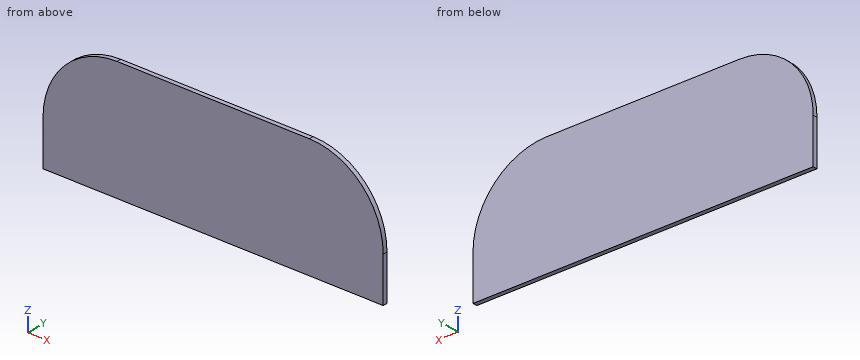
```python
from build123d import *

# Parameters (mm, degrees)
F1_DEPTH = 0.3


with BuildPart() as f1:
    # F0 (on Front) → F1 (new body)
    with BuildSketch(Plane.XZ):
        with BuildLine():
            Line((0, 3), (0, 0))
            Line((0, 0), (23, 0))
            Line((23, 0), (23, 3))
            ThreePointArc((23, 3), (21.535534, 6.535534), (18, 8))
            Line((18, 8), (5, 8))
            ThreePointArc((5, 8), (1.464466, 6.535534), (0, 3))
        make_face()
    extrude(amount=F1_DEPTH)


solid = f1.part
```
Check sheet for the modelled part. Datum: model origin and axes. Units: mm. Coordinates: 2 decimals unless noted, no trailing zeros. Loops run counter-clockwise (first coordinate to the right, second up) from the corner with the lowest first, then second, coordinate; pieces in that order, holes last.
1) Material ranges on probe 1 along Z at (x, y) = (1.5, -0.05); probe 2 along Z at (x, y) = (19.75, -0.2); probe 3 along X at (y, z) = (-0.15, 4.5), recorded low to high.
2) Sectioned sample at A-A (y = -0.05). Record the boundary of the cut face in (x, z), and give its area (3 significant figures).
3) Sectioned sample at B-B (z = 5). Record the boundary of the cut face in (x, y).
4) Sectioned sample at C-C (x = 3). Record the boundary of the cut face in (y, z), and give its area (3 significant figures).
Check sheet entries:
1. probe 1: z = 0 to 6.57
1. probe 2: z = 0 to 7.68
1. probe 3: x = 0.23 to 22.77
2. outline: (0, 0) - (23, 0) - (23, 3) arc R5 ccw to (18, 8) - (5, 8) arc R5 ccw to (0, 3) - close
2. area: 173 mm2
3. outline: (0.42, -0.3) - (22.58, -0.3) - (22.58, 0) - (0.42, 0) - close
4. outline: (-0.3, 0) - (0, 0) - (0, 7.58) - (-0.3, 7.58) - close
4. area: 2.27 mm2
